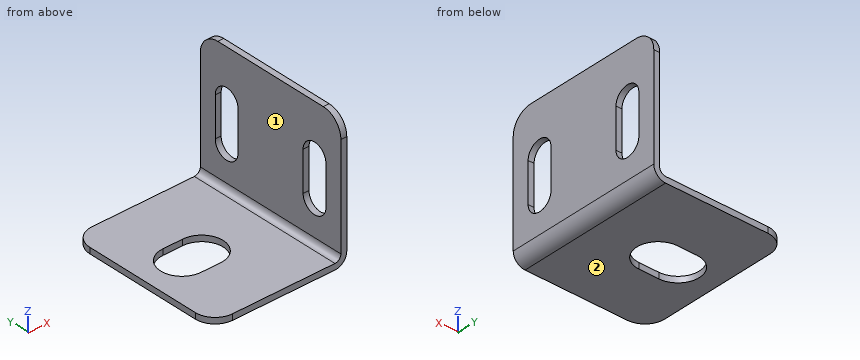
```python
from build123d import *

# Parameters (mm, degrees)
SKETCH1_W                = 33.02
SKETCH1_H                = 20.32
BOSS_EXTRUDE1_DEPTH      = 0.75946
M3_SLOTS_REACH           = 24.731
M5_SLOT_REACH            = 24.731
FILLET1_R                = 2.54
SKETCHED_START           = -3.237390165
SKETCHED_BEND1_OUTLINE_W = 20.32
SKETCHED_BEND1_OUTLINE_H = 0.75946
SKETCHED_BEND1_DEPTH     = 15.937390165
SKETCHED_START_2         = -3.83615356
SKETCHED_BEND1_2_DEPTH   = 0.10270916
SKETCHED_START_3         = -4.59815356
SKETCHED_BEND1_3_DEPTH   = 1.52146
SKETCHED_START_4         = -10.16
SKETCHED_BEND1_4_DEPTH   = 20.32


with BuildPart() as part:
    # Sketch1 → Boss-Extrude1 (new body)
    with BuildSketch(Plane.XY):
        with Locations((-3.81, 0)):
            Rectangle(SKETCH1_W, SKETCH1_H)
    extrude(amount=BOSS_EXTRUDE1_DEPTH)

    # Sketch4 → M3 Slots (cut, up to next)
    with BuildSketch(Plane.XY.offset(0.75946), mode=Mode.PRIVATE) as m3_slots_sk1:
        with BuildLine():
            Line((1.27, 8), (6.35, 8))
            ThreePointArc((6.35, 8), (8, 6.35), (6.35, 4.7))
            Line((6.35, 4.7), (1.27, 4.7))
            ThreePointArc((1.27, 4.7), (-0.38, 6.35), (1.27, 8))
        make_face()
    m3_slots_tool1 = extrude(m3_slots_sk1.sketch, amount=-M3_SLOTS_REACH, mode=Mode.PRIVATE) & part.part
    # Sketch4 → M3 Slots (cut, up to next)
    with BuildSketch(Plane.XY.offset(0.75946), mode=Mode.PRIVATE) as m3_slots_sk2:
        with BuildLine():
            Line((1.27, -4.7), (6.35, -4.7))
            ThreePointArc((6.35, -4.7), (8, -6.35), (6.35, -8))
            Line((6.35, -8), (1.27, -8))
            ThreePointArc((1.27, -8), (-0.38, -6.35), (1.27, -4.7))
        make_face()
    m3_slots_tool2 = extrude(m3_slots_sk2.sketch, amount=-M3_SLOTS_REACH, mode=Mode.PRIVATE) & part.part
    add(m3_slots_tool1.solids().sort_by_distance((3.81, 6.35, 0.75946))[0], mode=Mode.SUBTRACT)
    add(m3_slots_tool2.solids().sort_by_distance((3.81, -6.35, 0.75946))[0], mode=Mode.SUBTRACT)

    # Sketch5 → M5 Slot (cut, up to next)
    with BuildSketch(Plane.XY.offset(0.75946), mode=Mode.PRIVATE) as m5_slot_sk1:
        with BuildLine():
            Line((-15.24, 2.75), (-12.7, 2.75))
            ThreePointArc((-12.7, 2.75), (-9.95, 0), (-12.7, -2.75))
            Line((-12.7, -2.75), (-15.24, -2.75))
            ThreePointArc((-15.24, -2.75), (-17.99, 0), (-15.24, 2.75))
        make_face()
    m5_slot_tool1 = extrude(m5_slot_sk1.sketch, amount=-M5_SLOT_REACH, mode=Mode.PRIVATE) & part.part
    add(m5_slot_tool1.solids().sort_by_distance((-13.97, 0, 0.75946))[0], mode=Mode.SUBTRACT)

    # Fillet1
    fillet1_edges = [part.edges().sort_by_distance(p)[0] for p in [
        (-20.32, -10.16, 0.37973),
        (-20.32, 10.16, 0.37973),
        (12.7, 10.16, 0.37973),
        (12.7, -10.16, 0.37973),
    ]]
    fillet(fillet1_edges, radius=FILLET1_R)

    # Sketched Bend1: read off the stored shape, not the designer's step
    # Sketched Bend1 outline → Sketched Bend1 (cut)
    with BuildSketch(Plane.YZ.offset(SKETCHED_START)):
        with Locations((0, 0.37973)):
            Rectangle(SKETCHED_BEND1_OUTLINE_W, SKETCHED_BEND1_OUTLINE_H)
    extrude(amount=SKETCHED_BEND1_DEPTH, mode=Mode.SUBTRACT)

    # Sketched Bend1 2 outline → Sketched Bend1 2 (add)
    with BuildSketch(Plane.YZ.offset(SKETCHED_START_2)):
        with BuildLine():
            Line((7.62, 17.24330644), (-7.62, 17.24330644))
            ThreePointArc((-7.62, 17.24330644), (-9.416051224, 16.499357664), (-10.16, 14.70330644))
            Line((-10.16, 14.70330644), (-10.16, 0.75946))
            Line((-10.16, 0.75946), (10.16, 0.75946))
            Line((10.16, 0.75946), (10.16, 14.70330644))
            ThreePointArc((10.16, 14.70330644), (9.416051224, 16.499357664), (7.62, 17.24330644))
        make_face()
        with BuildLine():
            ThreePointArc((-8, 10.89330644), (-6.35, 12.54330644), (-4.7, 10.89330644))
            Line((-4.7, 10.89330644), (-4.7, 5.81330644))
            ThreePointArc((-4.7, 5.81330644), (-6.35, 4.16330644), (-8, 5.81330644))
            Line((-8, 5.81330644), (-8, 10.89330644))
        make_face(mode=Mode.SUBTRACT)
        with BuildLine():
            ThreePointArc((4.7, 10.89330644), (6.35, 12.54330644), (8, 10.89330644))
            Line((8, 10.89330644), (8, 5.81330644))
            ThreePointArc((8, 5.81330644), (6.35, 4.16330644), (4.7, 5.81330644))
            Line((4.7, 5.81330644), (4.7, 10.89330644))
        make_face(mode=Mode.SUBTRACT)
    extrude(amount=SKETCHED_BEND1_2_DEPTH)

    # Sketched Bend1 3 outline → Sketched Bend1 3 (add)
    with BuildSketch(Plane.YZ.offset(SKETCHED_START_3)):
        with BuildLine():
            Line((7.62, 17.24330644), (-7.62, 17.24330644))
            ThreePointArc((-7.62, 17.24330644), (-9.416051224, 16.499357664), (-10.16, 14.70330644))
            Line((-10.16, 14.70330644), (-10.16, 0.75946))
            Line((-10.16, 0.75946), (10.16, 0.75946))
            Line((10.16, 0.75946), (10.16, 14.70330644))
            ThreePointArc((10.16, 14.70330644), (9.416051224, 16.499357664), (7.62, 17.24330644))
        make_face()
        with BuildLine():
            ThreePointArc((-8, 10.89330644), (-6.35, 12.54330644), (-4.7, 10.89330644))
            Line((-4.7, 10.89330644), (-4.7, 5.81330644))
            ThreePointArc((-4.7, 5.81330644), (-6.35, 4.16330644), (-8, 5.81330644))
            Line((-8, 5.81330644), (-8, 10.89330644))
        make_face(mode=Mode.SUBTRACT)
        with BuildLine():
            ThreePointArc((4.7, 10.89330644), (6.35, 12.54330644), (8, 10.89330644))
            Line((8, 10.89330644), (8, 5.81330644))
            ThreePointArc((8, 5.81330644), (6.35, 4.16330644), (4.7, 5.81330644))
            Line((4.7, 5.81330644), (4.7, 10.89330644))
        make_face(mode=Mode.SUBTRACT)
    extrude(amount=SKETCHED_BEND1_3_DEPTH)

    # Sketched Bend1 4 outline → Sketched Bend1 4 (cut)
    with BuildSketch(Plane(origin=(0, 0, 0), x_dir=(1, 0, 0), z_dir=(0, 1, 0)).offset(SKETCHED_START_4)):
        with BuildLine():
            Line((-4.59815356, -17.24330644), (-3.83615356, -17.24330644))
            Line((-3.83615356, -17.24330644), (-3.83615356, -1.52146))
            ThreePointArc((-3.83615356, -1.52146), (-4.059338193, -0.982644633), (-4.59815356, -0.75946))
            Line((-4.59815356, -0.75946), (-4.59815356, -17.24330644))
        make_face()
        with BuildLine():
            ThreePointArc((-4.59815356, 0), (-3.522318877, -0.445625317), (-3.07669356, -1.52146))
            Line((-3.07669356, -1.52146), (-3.07669356, -0.75946))
            Line((-3.07669356, -0.75946), (-3.237390165, -0.75946))
            Line((-3.237390165, -0.75946), (-3.237390165, 0))
            Line((-3.237390165, 0), (-4.59815356, 0))
        make_face()
    extrude(amount=SKETCHED_BEND1_4_DEPTH, mode=Mode.SUBTRACT)


solid = part.part
```
Could you check a few things on this model? Use its own coordinates, in mm. Face numbers are marked on the shaded views. A direction names the side the tool comes from. Round coordinates to 2 decimals unless told otherwise and drop trailing zeros. Write each loop counter-clockwise with the first axis right and the second up, starting at its lowest first coordinate (ties: lowest second). Pieces come first, ordered by that corner, then holes.
(1) If I drill on probe 1 along Z at (x, y) = (-14.5, -7.75); probe 2 along X at (y, z) = (-8.75, 6.25); probe 3 along Z at (x, y) = (-4, -6), over which ranges is the centre line in solid material (lowest first)?
Findings below:
probe 1: z = 0 to 0.76
probe 2: x = -3.84 to -3.08
probe 3: z = 0.12 to 1.05
(2) Suppose I cut it at C-C on y = 6.35. Write out the boundary of the cut face in (x, z), and give its area (3 significant figures).
Findings below:
outline: (-20.32, 0) - (-4.6, 0) arc R1.52 ccw to (-3.08, 1.52) - (-3.08, 4.16) - (-3.84, 4.16) - (-3.84, 1.52) arc R0.76 cw to (-4.6, 0.76) - (-20.32, 0.76) - close; (-3.84, 12.54) - (-3.08, 12.54) - (-3.08, 17.24) - (-3.84, 17.24) - close
area: 18.9 mm2
(3) Which directions (+Z, -Z, +X, -X, +Y, -Y) give clear straight access to the entire face, cutting with the end or side of a thin tool? Please do the marked faces 1 and 2.
Findings below:
face 1: +Z, -X, +Y, -Y
face 2: -Z, +X, -X, +Y, -Y
(4) Suppose I cut it at A-A on z = 10. Write out the boundary of the cut face in (x, y), and give its area (3 significant figures).
Findings below:
outline: (-3.84, -10.16) - (-3.08, -10.16) - (-3.08, -8) - (-3.84, -8) - close; (-3.84, -4.7) - (-3.08, -4.7) - (-3.08, 4.7) - (-3.84, 4.7) - close; (-3.84, 8) - (-3.08, 8) - (-3.08, 10.16) - (-3.84, 10.16) - close
area: 10.4 mm2
(5) Suppose I cut it at B-B on x = -13. Write out the boundary of the cut face in (y, z), and give its area (3 significant figures).
Findings below:
outline: (-10.16, 0) - (-2.75, 0) - (-2.75, 0.76) - (-10.16, 0.76) - close; (2.75, 0) - (10.16, 0) - (10.16, 0.76) - (2.75, 0.76) - close
area: 11.3 mm2
(6) Suppose I cut it at D-D on y = -3.25. Write out the boundary of the cut face in (x, z).
Findings below:
outline: (-20.32, 0) - (-4.6, 0) arc R1.52 ccw to (-3.08, 1.52) - (-3.08, 17.24) - (-3.84, 17.24) - (-3.84, 1.52) arc R0.76 cw to (-4.6, 0.76) - (-20.32, 0.76) - close
(7) For pin 1 (5 mm diameter, centred on x = -8.5, y = -7, fed in from +Z); pin 2 (5 mm diameter, centred on x = -7, z = 11.5, fed in from +Y); pin 3 (1.5 mm diameter, centred on y = 1, z = 13, fed in from -X), each with a flat end and sliding along its axis, tell me the tip position at first contact or that it passes through.
Findings below:
pin 1: stops at z = 0.76
pin 2: passes through
pin 3: stops at x = -3.84
